Check sheet for the modelled part. Datum: model origin and axes. Units: mm. Round coordinates to 2 decimals unless told otherwise and drop trailing zeros. Write each loop counter-clockwise with the first axis right and the second up, starting at its lowest first coordinate (ties: lowest second). Pieces come first, ordered by that corner, then holes.
Item 1: Section check B-B, the plane z = 22.5. Record the cut outline in (x, y).
Item 2: Depth check by flat-ended pin: pin 1 (3 mm diameter, centred on y = -17.5, z = 15.5, fed in from +X); pin 2 (12 mm diameter, centred on x = -2.5, y = -11.5, fed in from -Z); pin 3 (1.5 mm diameter, centred on x = -20, z = 22, fed in from +Y); pin 4 (5 mm diameter, centred on x = -19.5, y = 14.5, fed in from +Z). Enter the tip coordinate at first touch or a pass-through.
Item 3: Section check A-A, the plane z = 10.75. Record the cut outline in (x, y), plus the area to 3 significant figures.
Item 4: Material ranges on line 1 along X through (y, z) = (-21, 12); line 2 along Y through (x, z) = (8, 16); line 3 along X through (y, z) = (-21.5, 19.5), recorded low to high.
Item 5: Section check C-C, the plane z = 4. Record the cut outline in (x, y), plus the area to 3 significant figures.
from build123d import *

# Parameters (mm, degrees)
F1_DEPTH = 25.4


# Not quite as in the source:
# - a fillet or chamfer that OpenCascade refuses, or shapes differently, is made with other operations: its cross-section is extruded or revolved along the edge and cut away or added


with BuildPart() as f1:
    # F0 (on Top) → F1 (new body)
    with BuildSketch(Plane.XY):
        with BuildLine():
            Line((0, 0), (25.6860326238, 0))
            ThreePointArc((25.6860326238, 0), (18.1627678501, 18.1627678501), (0, 25.6860326238))
            Line((0, 25.6860326238), (0, 0))
        make_face()
        with BuildLine():
            ThreePointArc((0, -25.6860326238), (18.1627678501, -18.1627678501), (25.6860326238, 0))
            Line((25.6860326238, 0), (0, 0))
            Line((0, 0), (0, -25.6860326238))
        make_face()
        with BuildLine():
            ThreePointArc((-25.6860326238, 0), (-18.1627678501, -18.1627678501), (0, -25.6860326238))
            Line((0, -25.6860326238), (0, 0))
            Line((0, 0), (-25.6860326238, 0))
        make_face()
        with BuildLine():
            Line((0, 0), (0, 25.6860326238))
            ThreePointArc((0, 25.6860326238), (-18.1627678501, 18.1627678501), (-25.6860326238, 0))
            Line((-25.6860326238, 0), (0, 0))
        make_face()
    extrude(amount=F1_DEPTH)

    # F2: fillet of radius 5.08 on 3 edges, made by hand

    # F2_s1 → F2_t2 (revolve, cut)
    with BuildSketch(Plane.YZ):
        with BuildLine():
            ThreePointArc((25.6864326238, 20.3190343146), (24.1981350723, 23.9121024484), (20.6050669384, 25.4004))
            Line((20.6050669384, 25.4004), (20.6050669384, 25.9085365685))
            ThreePointArc((20.6050669384, 25.9085365685), (23.1455497811, 25.9081365685), (25.6860326238, 25.9081365685))
            Line((25.6860326238, 25.9081365685), (26.1941691924, 25.4))
            ThreePointArc((26.1941691924, 25.4), (26.1941691924, 22.8595171573), (26.1945691924, 20.3190343146))
            Line((26.1945691924, 20.3190343146), (25.6864326238, 20.3190343146))
        make_face()
    revolve(axis=Axis((0, 0, 25.4), (0, 0, 1)), mode=Mode.SUBTRACT)

    # F2_s3 → F2_t4 (revolve, cut)
    with BuildSketch(Plane.YZ):
        with BuildLine():
            ThreePointArc((25.6864326238, 5.0809656854), (24.1981350723, 1.4878975516), (20.6050669384, -0.0004))
            Line((20.6050669384, -0.0004), (20.6050669384, -0.5085365685))
            ThreePointArc((20.6050669384, -0.5085365685), (23.1455497811, -0.5081365685), (25.6860326238, -0.5081365685))
            Line((25.6860326238, -0.5081365685), (26.1941691924, 0))
            ThreePointArc((26.1941691924, 0), (26.1941691924, 2.5404828427), (26.1945691924, 5.0809656854))
            Line((26.1945691924, 5.0809656854), (25.6864326238, 5.0809656854))
        make_face()
    revolve(axis=Axis((0, 0, 0), (0, 0, 1)), mode=Mode.SUBTRACT)


solid = f1.part
Values found:
1. outline: circle Ø50.39 at (0, 0)
2. pin 1: stops at x = 20.09
2. pin 2: stops at z = 0
2. pin 3: stops at y = 16.65
2. pin 4: stops at z = 25.26
3. outline: circle Ø51.37 at (0, 0)
3. area: 2,070 mm2
4. line 1: x = -14.79 to 14.79
4. line 2: y = -24.41 to 24.41
4. line 3: x = -14.05 to 14.05
5. outline: circle Ø51.14 at (0, 0)
5. area: 2,050 mm2
